```python
from build123d import *

# Parameters (mm, degrees)
F0_R     = 2.5
F1_DEPTH = 1.25


with BuildPart() as f1:
    # F0 (on Top) → F1 (new body, symmetric)
    with BuildSketch(Plane.XY):
        with BuildLine():
            Line((40, -40), (40, 40))
            Line((40, 40), (-40, 40))
            Line((-40, 40), (-40, -40))
            Line((-40, -40), (-1, -40))
            Line((-1, -40), (-1, -21.5))
            Line((-1, -21.5), (-1, -21.476732))
            ThreePointArc((-1, -21.476732), (-14.845033, 15.552331), (21.5, 0))
            ThreePointArc((21.5, 0), (15.552331, -14.845033), (1, -21.476732))
            Line((1, -21.476732), (1, -21.5))
            Line((1, -21.5), (1, -40))
            Line((1, -40), (40, -40))
        make_face()
        with Locations((-35, -31)):
            Circle(F0_R, mode=Mode.SUBTRACT)
        with Locations((35, -31)):
            Circle(F0_R, mode=Mode.SUBTRACT)
        with Locations((-35, 31)):
            Circle(F0_R, mode=Mode.SUBTRACT)
        with Locations((35, 31)):
            Circle(F0_R, mode=Mode.SUBTRACT)
    extrude(amount=F1_DEPTH, both=True)


solid = f1.part
```
Can you work these out from the model? Positions are in its coordinate system, mm. A direction names the side the tool comes from. Give positions to 0.01 mm unless a question says otherwise; leave off trailing zeros. Loops run counter-clockwise (first coordinate to the right, second up) from the corner with the lowest first, then second, coordinate; pieces in that order, holes last. Notation, with made-up numbers: M -16,13.25 L 28,13.25 A23 ccw 28,36.25 Z; hole C -3.75,87.25 d1. An arc over 180 degrees is marked long. Use one line per item in the form item = value. Start each with the question number.
(1) I want a section at D-D, the plane x = 13.5. Write out the boundary of the cut face in (y, z).
(2) Please list where these lines run through material, in increasing order: line 1 (Y direction, x = 35, z = 0.55); line 2 (X direction, y = -36, z = -0.75); line 3 (Y direction, x = -34, z = -0.55).
(3) I want a section at A-A, the plane y = -35. Write out the boundary of the cut face in (x, z), and give its area (3 significant figures).
(4) Thinking about a two-plate mould opening in Y: for faces 1 (the flat face through (-21, -40, 0)), 2 (the cylindrical face through (36.34, 33.11, -0.02)), 3 (the flat face through (1, -31, 0)), which applies, released by +Y, released by -Y, zero draft, split by the parting line, or undercut?
(5) I'm going to push a flat-ended pin straight in: P1, Ø4.5, axis at x = -35, y = 31, coming from the +Z side. Where does the tip first touch, or does it pass through?
(6) I want a section at C-C, the plane z = 0.2. Write out the boundary of the cut face in (x, y).
(7) On a 3-axis mill with a long thin cutter (end or side, diameter ignored), from which of +Z, -Z, +X, -X, +Y, -Y can I reach the whole of each face in a straight line? I mean faces 4 (the flat face through (-1, -31, 0)), 5 (the flat face through (-40, 1, 0)). Say none if no direction works.
(8) I want a section at B-B, the plane x = -35. Write out the boundary of the cut face in (y, z), and give its area (3 significant figures).
Worked out:
q1.outline = M -40,-1.25 L -16.73,-1.25 L -16.73,1.25 L -40,1.25 Z; M 16.73,-1.25 L 40,-1.25 L 40,1.25 L 16.73,1.25 Z
q2.line_1 = -40 to -33.5, -28.5 to 28.5, 33.5 to 40
q2.line_2 = -40 to -1, 1 to 40
q2.line_3 = -40 to -33.29, -28.71 to 28.71, 33.29 to 40
q3.outline = M -40,-1.25 L -1,-1.25 L -1,1.25 L -40,1.25 Z; M 1,-1.25 L 40,-1.25 L 40,1.25 L 1,1.25 Z
q3.area = 195 mm²
q4.face_1 = released by -Y
q4.face_2 = undercut
q4.face_3 = zero draft
q5.P1 = through
q6.outline = M -40,-40 L -1,-40 L -1,-21.48 A21.5 cw long 1,-21.48 L 1,-40 L 40,-40 L 40,40 L -40,40 Z; hole C -35,-31 d5; hole C -35,31 d5; hole C 35,-31 d5; hole C 35,31 d5
q7.face_4 = +Z, -Z, -Y
q7.face_5 = +Z, -Z, -X, +Y, -Y
q8.outline = M -40,-1.25 L -33.5,-1.25 L -33.5,1.25 L -40,1.25 Z; M -28.5,-1.25 L 28.5,-1.25 L 28.5,1.25 L -28.5,1.25 Z; M 33.5,-1.25 L 40,-1.25 L 40,1.25 L 33.5,1.25 Z
q8.area = 175 mm²
